Work out the finished part from the listing and answer in its coordinate system (mm). Give positions to 0.01 mm unless a question says otherwise; leave off trailing zeros. Loops run counter-clockwise (first coordinate to the right, second up) from the corner with the lowest first, then second, coordinate; pieces in that order, holes last. Notation, with made-up numbers: (29.25, 73.25) - (36.25, 73.25) arc R18 cw to (36.25, 94.25) - close; hole circle Ø11 at (55.25, -16.5). An arc over 180 degrees is marked (long way). One line per question, with ' | ' between items. Start each with the question number.
1. Section B-B (x = 0) is taken. Determine the outline of the cut face in (y, z).
2. For a pull along X with two mould halves and no side action, classify faces 1 (the face through (7.39, -64.14, 6.46)), 2 (the face through (-7.14, -64.1, 6.46)), 3 (the face through (0, 6.928, 6)), 4 (the face through (0, 2, 6)) as released by +X, released by -X, zero draft, split by the parting line, or undercut.
3. Find the intervals of material crossed by line 1 (Y direction, x = 0, z = 7); line 2 (X direction, y = -1.5, z = 6.5); line 3 (X direction, y = -51, z = 11.25), in increasing order.
4. Section A-A (z = 8.25) is taken. Determine the outline of the cut face in (x, y).
5. Each of these flat-tipped pins is pushed along its axis until it touches: pin 1 (1 mm diameter, centred on y = -3.5, z = 2.5, fed in from +X); pin 2 (6 mm diameter, centred on y = -35.5, z = 3, fed in from +X). Where does it stop, or does it pass through?
Autodesk Inventor part; units mm, degrees
ref_plane "YZ Plane" through (0, 0, 0) normal (1, 0, 0) x (0, 1, 0)
ref_plane "XZ Plane" through (0, 0, 0) normal (0, 1, 0) x (-1, 0, 0)
ref_plane "XY Plane" through (0, 0, 0) normal (0, 0, 1) x (1, 0, 0)
sketch "Sketch1" plane through (0, 0, 0) normal (0, 0, 1) x (1, 0, 0)
  circle A0 centre (0, 0) radius 2
  line L0 (-8, 0) -> (-8, -65)
  line L1 (-8, -65) -> (8.3, -65)
  line L2 (8.3, -65) -> (8, 0)
  line L3 (-8, 0) -> (-4, 6.9282)
  line L4 (-4, 6.9282) -> (4, 6.9282)
  line L5 (4, 6.9282) -> (8, 0)
  dimension "d0" = 4
  dimension "d2" = 65
  dimension "d3" = 16.3
extrude "Extrusion1" add sketch "Sketch1" along normal blind 12.75
fillet "Fillet1" radius 1 4 edges at (-4, 6.9282, 6.375) (4, 6.9282, 6.375) (8, 0, 6.375) (-8, 0, 6.375)
fillet "Fillet2" radius 3 2 edges at (8.3, -65, 6.375) (-8, -65, 6.375)
properties part number "real arm"
Conclusion:
1) outline: (-65, 0) - (-2, 0) - (-2, 12.75) - (-65, 12.75) - close; (2, 0) - (6.93, 0) - (6.93, 12.75) - (2, 12.75) - close
2) face 1: released by +X | face 2: released by -X | face 3: zero draft | face 4: undercut
3) line 1: -65 to -2, 2 to 6.93 | line 2: -8 to -1.32, 1.32 to 8.01 | line 3: -8 to 8.24
4) outline: (-8, -62) arc R3 ccw to (-5, -65) - (5.29, -65) arc R3 ccw to (8.29, -61.99) - (8, -0.27) arc R1 ccw to (7.87, 0.23) - (4.29, 6.43) arc R1 ccw to (3.42, 6.93) - (-3.42, 6.93) arc R1 ccw to (-4.29, 6.43) - (-7.87, 0.23) arc R1 ccw to (-8, -0.27) - close; hole circle Ø4 at (0, 0)
5) pin 1: x = 8.02 | pin 2: x = 8.18
